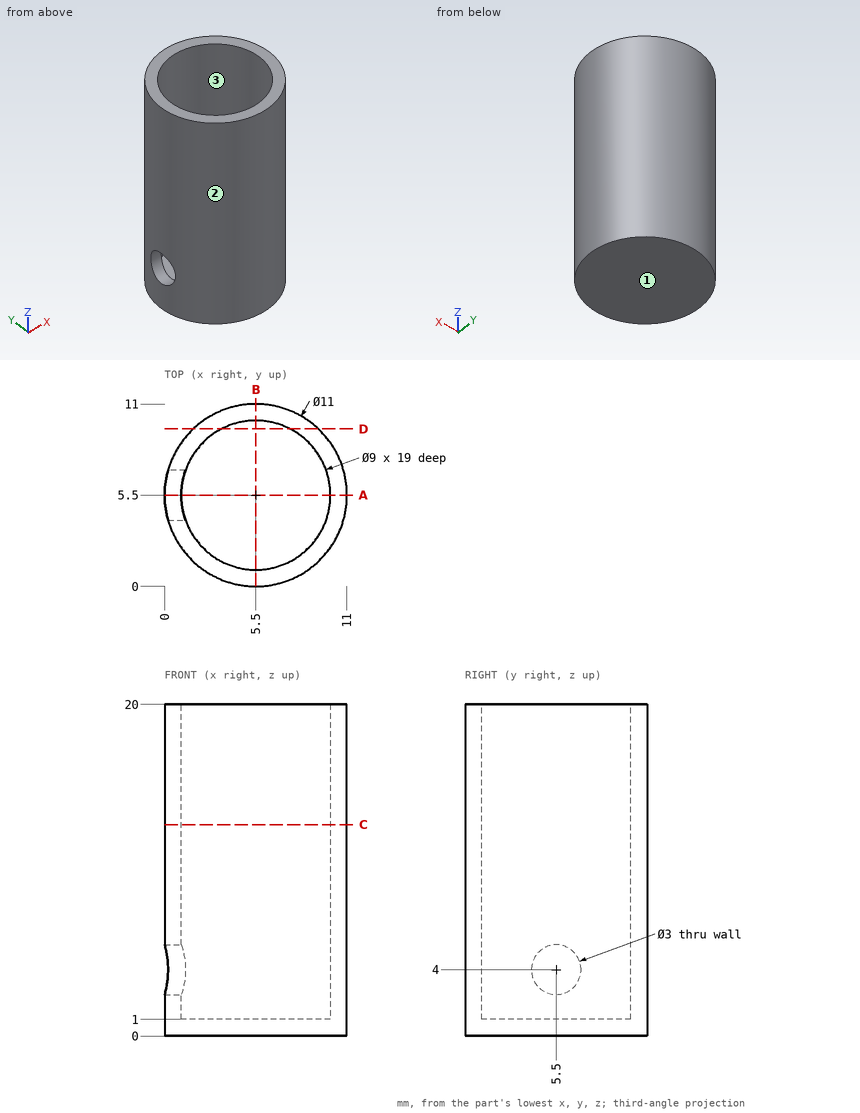
Here's the drawing with two shaded views (mm, measured from the low corner). I have some questions. Round coordinates to 2 decimals unless told otherwise and drop trailing zeros. Loops run counter-clockwise (first coordinate to the right, second up) from the corner with the lowest first, then second, coordinate; pieces in that order, holes last. Notation, with made-up numbers: (-19, -33.75) - (1, -33.75) arc R21 ccw to (1, 3.25) - close; hole circle Ø9 at (86.5, 46). An arc over 180 degrees is marked (long way). Write item = value, one per line.
1) I'm going to push flat-ended pins straight in: P1, Ø3, axis at y = 8.5, z = 17, coming from the -X side; P2, Ø6, axis at x = 9.5, z = 6, coming from the -Y side; P3, Ø1.5, axis at y = 3.5, z = 8, coming from the -X side. Where does each tip first touch, or does it pass through?
Computed:
P1 = 0.21
P2 = 0.09
P3 = 0.14
2) Imagine slicing it at D-D (y = 9.5). Please give me the cut outline in (x, z).
Computed:
outline = (1.73, 0) - (9.27, 0) - (9.27, 20) - (7.56, 20) - (7.56, 1) - (3.44, 1) - (3.44, 20) - (1.73, 20) - close
3) If we mould it in two halves opening along X, with no side actions, what happens to the marked faces 1, 2 and 3? For each: pulls with the +X half, pulls with the -X half, needs draft (parallel to the pull), parting line crosses it, or undercut.
Computed:
face_1 = needs draft
face_2 = parting line crosses it
face_3 = undercut
4) Imagine slicing it at B-B (x = 5.5). Please give me the cut outline in (y, z).
Computed:
outline = (0, 0) - (11, 0) - (11, 20) - (10, 20) - (10, 1) - (1, 1) - (1, 20) - (0, 20) - close
5) I need wall thicknesses on line 1 along Z through (x, y) = (4.25, 3); line 2 along Y through (x, z) = (5.5, 14.5); line 3 along Y through (x, z) = (8.5, 19.25). Which ranges of each line are inside material? Lowest first, please. Write a range as from..to.
Computed:
line_1 = 0..1
line_2 = 0..1, 10..11
line_3 = 0.89..2.15, 8.85..10.11
6) Imagine slicing it at C-C (z = 12.75). Please give me the cut outline in (x, y), and give its area (3 significant figures).
Computed:
outline = circle Ø11 at (5.5, 5.5); hole circle Ø9 at (5.5, 5.5)
area = 31.4 mm2
7) Imagine slicing it at A-A (y = 5.5). Please give me the cut outline in (x, z).
Computed:
outline = (0, 0) - (11, 0) - (11, 20) - (10, 20) - (10, 1) - (1, 1) - (1, 2.5) - (0, 2.5) - close; (0, 5.5) - (1, 5.5) - (1, 20) - (0, 20) - close
